Work out the finished part from the listing and answer in its coordinate system (mm). Round coordinates to 2 decimals unless told otherwise and drop trailing zeros. Write each loop counter-clockwise with the first axis right and the second up, starting at its lowest first coordinate (ties: lowest second). Pieces come first, ordered by that corner, then holes. Notation, with made-up numbers: (82, 29) - (108, 29) arc R10 cw to (108, 46) - close; hole circle Ø9 at (50.25, -36). An arc over 180 degrees is marked (long way). Write item = value, one per line. Start each with the question number.
from build123d import *

# Parameters (mm, degrees)
SKETCH1_W           = 88.9
SKETCH1_H           = 44.45
BOSS_EXTRUDE1_DEPTH = 3.175
CUT_EXTRUDE1_DEPTH  = 50.797929174
SKETCH7_W           = 12.7
SKETCH7_H           = 19.05
CUT_EXTRUDE2_DEPTH  = 50.797929174


with BuildPart() as part:
    # Sketch1 → Boss-Extrude1 (new body)
    with BuildSketch(Plane(origin=(0, 0, 0), x_dir=(1, 0, 0), z_dir=(0, 1, 0))):
        Rectangle(SKETCH1_W, SKETCH1_H)
    extrude(amount=BOSS_EXTRUDE1_DEPTH)

    # Sketch3 → Cut-Extrude1 (cut, through all)
    with BuildSketch(Plane.XZ):
        with BuildLine():
            Line((-22.9888034, 11.2), (-29.3388034, 11.2))
            ThreePointArc((-29.3388034, 11.2), (-31.0388034, 9.5), (-29.3388034, 7.8))
            Line((-29.3388034, 7.8), (-22.9888034, 7.8))
            ThreePointArc((-22.9888034, 7.8), (-21.2888034, 9.5), (-22.9888034, 11.2))
        make_face()
        with BuildLine():
            Line((-30.950911086, 1.7), (-37.2763034, 1.7))
            ThreePointArc((-37.2763034, 1.7), (-38.9763034, 0), (-37.2763034, -1.7))
            Line((-37.2763034, -1.7), (-30.950911086, -1.7))
            ThreePointArc((-30.950911086, -1.7), (-31.2438034, 0), (-30.950911086, 1.7))
        make_face()
        with BuildLine():
            Line((-21.376695714, 1.7), (-30.950911086, 1.7))
            ThreePointArc((-30.950911086, 1.7), (-31.2438034, 0), (-30.950911086, -1.7))
            Line((-30.950911086, -1.7), (-21.376695714, -1.7))
            ThreePointArc((-21.376695714, -1.7), (-21.157561943, -0.86252332), (-21.0838034, 0))
            ThreePointArc((-21.0838034, 0), (-21.157561943, 0.86252332), (-21.376695714, 1.7))
        make_face()
        with BuildLine():
            ThreePointArc((-21.376695714, 1.7), (-26.1638034, 5.08), (-30.950911086, 1.7))
            Line((-30.950911086, 1.7), (-21.376695714, 1.7))
        make_face()
        with BuildLine():
            Line((-15.0513034, 1.7), (-21.376695714, 1.7))
            ThreePointArc((-21.376695714, 1.7), (-21.157561943, 0.86252332), (-21.0838034, 0))
            ThreePointArc((-21.0838034, 0), (-21.157561943, -0.86252332), (-21.376695714, -1.7))
            Line((-21.376695714, -1.7), (-15.0513034, -1.7))
            ThreePointArc((-15.0513034, -1.7), (-13.3513034, 0), (-15.0513034, 1.7))
        make_face()
        with BuildLine():
            Line((-21.376695714, -1.7), (-30.950911086, -1.7))
            ThreePointArc((-30.950911086, -1.7), (-26.1638034, -5.08), (-21.376695714, -1.7))
        make_face()
        with BuildLine():
            Line((-29.3388034, -11.2), (-22.9888034, -11.2))
            ThreePointArc((-22.9888034, -11.2), (-21.2888034, -9.5), (-22.9888034, -7.8))
            Line((-22.9888034, -7.8), (-29.3388034, -7.8))
            ThreePointArc((-29.3388034, -7.8), (-31.0388034, -9.5), (-29.3388034, -11.2))
        make_face()
    cut_extrude1 = extrude(amount=-CUT_EXTRUDE1_DEPTH, mode=Mode.SUBTRACT)

    # Mirror1: Cut-Extrude1 across plane
    add(cut_extrude1.mirror(Plane(origin=(0, 0, 0), x_dir=(0, 0, 1), z_dir=(1, 0, 0))), mode=Mode.SUBTRACT)

    # Sketch7 → Cut-Extrude2 (cut, through all)
    with BuildSketch(Plane(origin=(0, 3.175, 0), x_dir=(1, 0, 0), z_dir=(0, 1, 0))):
        with Locations((0, 12.7)):
            Rectangle(SKETCH7_W, SKETCH7_H)
    extrude(amount=-CUT_EXTRUDE2_DEPTH, mode=Mode.SUBTRACT)


solid = part.part
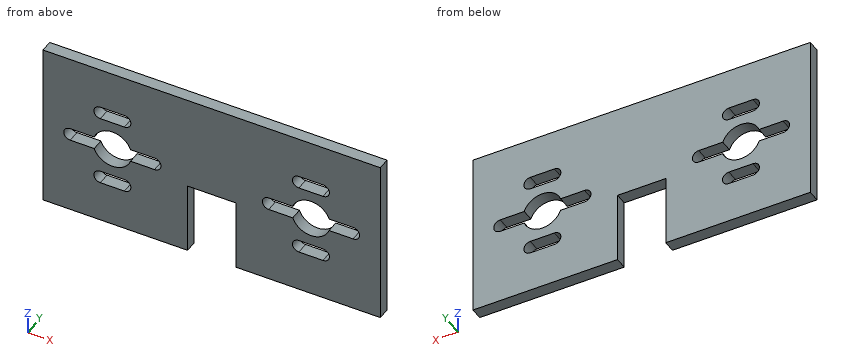
1. Find section D-D on y = 1.7. Give the number of separate pieces and of enclosed holes in the cut face, plus the area to 3 significant figures.
2. Consider line 1 (X direction, y = 2.15, z = 9); line 2 (X direction, y = 1.6, z = -5.5); line 3 (X direction, y = 1.75, z = -10). Determine where each line is inside the solid, lowest interval first.
3. Find section B-B on z = 0. Give the vertices of the cut face in (x, y) (3 decimals), plus the area to 3 significant figures.
4. Find section C-C on z = 9.5. Give the vertices of the cut face in (x, y) (3 decimals).
5. Find section A-A on z = -9.5. Give the vertices of the cut face in (x, y) (3 decimals), plus the area to 3 significant figures.
Answer key:
q1.separate_pieces = 1
q1.enclosed_holes = 6
q1.area = 3,320 mm²
q2.line_1 = -44.45 to -30.96, -21.36 to 21.36, 30.96 to 44.45
q2.line_2 = -44.45 to -6.35, 6.35 to 44.45
q2.line_3 = -44.45 to -30.96, -21.36 to -6.35, 6.35 to 21.36, 30.96 to 44.45
q3.outline = (-44.45, 0) - (-38.976, 0) - (-38.976, 3.175) - (-44.45, 3.175) - close; (-13.351, 0) - (13.351, 0) - (13.351, 3.175) - (-13.351, 3.175) - close; (38.976, 0) - (44.45, 0) - (44.45, 3.175) - (38.976, 3.175) - close
q3.area = 120 mm²
q4.outline = (-44.45, 0) - (-31.039, 0) - (-31.039, 3.175) - (-44.45, 3.175) - close; (-21.289, 0) - (21.289, 0) - (21.289, 3.175) - (-21.289, 3.175) - close; (31.039, 0) - (44.45, 0) - (44.45, 3.175) - (31.039, 3.175) - close
q5.outline = (-44.45, 0) - (-31.039, 0) - (-31.039, 3.175) - (-44.45, 3.175) - close; (-21.289, 0) - (-6.35, 0) - (-6.35, 3.175) - (-21.289, 3.175) - close; (6.35, 0) - (21.289, 0) - (21.289, 3.175) - (6.35, 3.175) - close; (31.039, 0) - (44.45, 0) - (44.45, 3.175) - (31.039, 3.175) - close
q5.area = 180 mm²
